Autodesk Inventor part; units mm, degrees
ref_plane "YZ Plane" through (0, 0, 0) normal (1, 0, 0) x (0, 1, 0)
ref_plane "XZ Plane" through (0, 0, 0) normal (0, 1, 0) x (-1, 0, 0)
ref_plane "XY Plane" through (0, 0, 0) normal (0, 0, 1) x (1, 0, 0)
sketch "스케치1" plane through (0, 0, 0) normal (1, 0, 0) x (0, 1, 0)
  line L0 (0, 0) -> (50, 0)
  line L1 (50, 0) -> (50, -14)
  line L2 (50, -14) -> (0, -14)
  line L3 (0, -14) -> (0, 0)
  circle A0 centre (32, -7) radius 1.5
  circle A1 centre (3, -7) radius 1.5
  line L4 (60, 16.5) -> (50, 16.5)
  line L5 (50, 16.5) -> (50, -30.5)
  line L6 (50, -30.5) -> (60, -30.5)
  line L7 (60, -30.5) -> (60, 16.5)
  circle A2 centre (55, 11.5) radius 1.5
  circle A3 centre (55, -25.5) radius 1.5
  point P0 (50, -7)
  dimension "d0" = 50
  dimension "d1" = 14
  dimension "d2" = 3
  dimension "d3" = 3
  dimension "d4" = 29
  dimension "d5" = 7
  dimension "d6" = 7
  dimension "d10" = 3
  dimension "d11" = 10
  dimension "d12" = 47
  dimension "d13" = 3
  dimension "d14" = 3
  dimension "d15" = 37
  dimension "d16" = 5
  dimension "d17" = 5
  dimension "d18" = 5
extrude "돌출2" add sketch "스케치1" along normal blind 4
sketch "스케치2" plane through (4, 0, 0) normal (1, 0, 0) x (0, 0, -1)
  circle A0 centre (7, 3) radius 1.5
  circle A1 centre (7, 32) radius 1.5
  circle A2 centre (25.5, 55) radius 1.5
  circle A3 centre (-11.5, 55) radius 1.5
  line L0 (-16.5, 50) -> (0, 50)
  line L1 (0, 50) -> (0, 0)
  line L2 (0, 0) -> (14, 0)
  line L3 (14, 0) -> (14, 50)
  line L4 (14, 50) -> (30.5, 50)
  line L5 (30.5, 50) -> (30.5, 60)
  line L6 (30.5, 60) -> (-16.5, 60)
  line L7 (-16.5, 60) -> (-16.5, 50)
  line L8 (0, 50) -> (0, 0)
  line L9 (0, 42) -> (14, 42)
  line L10 (14, 0) -> (14, 50)
  dimension "d21" = 10
bend part "굽힘1" radius 10 angle 10 line through (4, 42, 0) along (0, 0, -1) centre toward (1, 0, 0) moving side (0, 1, 0) both sides no
properties part number "옆면PSD받침대" material "ABS 플라스틱"
Geometry: final body of the model. Coordinates: model frame, mm. A direction names the side the tool comes from. Give positions to 0.01 mm unless a question says otherwise; leave off trailing zeros. Loops run counter-clockwise (first coordinate to the right, second up) from the corner with the lowest first, then second, coordinate; pieces in that order, holes last. Notation, with made-up numbers: (-10, 48) -> (39, 48) arc R29 cw to (39, 86) -> close; hole circle Ø9 at (30.25, 68.5). An arc over 180 degrees is marked (long way). Put each result on its own line as item: value.
1. Cut plane C-C (z = -1.5). Return the cut outline in (x, y), plus the area to 3 significant figures.
Taken from the geometry:
outline: (0, 0) -> (4, 0) -> (4, 42) arc R10 cw to (4.15, 43.74) -> (6.97, 59.74) -> (3.04, 60.44) -> (0.21, 44.43) arc R14 ccw to (0, 42) -> close
area: 241 mm2
2. Cut plane B-B (z = -7). Return the cut outline in (x, y), plus the area to 3 significant figures.
Taken from the geometry:
outline: (0, 0) -> (4, 0) -> (4, 1.5) -> (0, 1.5) -> close; (0, 4.5) -> (4, 4.5) -> (4, 30.5) -> (0, 30.5) -> close; (0, 33.5) -> (4, 33.5) -> (4, 42) arc R10 cw to (4.15, 43.74) -> (6.97, 59.74) -> (3.04, 60.44) -> (0.21, 44.43) arc R14 ccw to (0, 42) -> close
area: 217 mm2
3. Pull-direction query (Y, two-part tool) for faces 1 (the cylindrical face through (4.04, 42.88, -6.9)), 2 (the flat face through (4, 55, 16.5)), 3 (the cylindrical face through (4.075, 54.98, -26.987)); classes: released by +Y, released by -Y, zero draft, split by the parting line, or undercut.
Taken from the geometry:
face 1: released by -Y
face 2: zero draft
face 3: undercut
4. Set-up query: faces 4 (the flat face through (3.24, 50.25, 8.37)), 5 (the flat face through (4, 21, -7)), 6 (the flat face through (3.24, 50.25, -22.13)), 7 (the flat face through (0, 21, -7)). Return all of +Z, -Z, +X, -X, +Y, -Y with unobstructed straight access to the full face (end or side cutting, diameter ignored); none if empty.
Taken from the geometry:
face 4: +Z, -X, -Y
face 5: +Z, -Z, +X, -Y
face 6: -Z, -X, -Y
face 7: +Z, -Z, -X, +Y, -Y
5. Pin query (flat end, axial travel): P1, Ø2, axis at x = 4.5, z = 11.5, coming from the -Y side; P2, Ø5, axis at y = 3, z = -7, coming from the +X side; P3, Ø2, axis at x = 2, z = 4.5, coming from the -Y side. Return the tip coordinate at first contact, or that it passes through.
Taken from the geometry:
P1: stops at y = 49.9
P2: stops at x = 4
P3: stops at y = 50.29
6. Cut plane D-D (y = 37). Return the cut outline in (x, z), plus the area to 3 significant figures.
Taken from the geometry:
outline: (0, -14) -> (4, -14) -> (4, 0) -> (0, 0) -> close
area: 56.0 mm2
7. Cut plane A-A (y = 3). Return the cut outline in (x, z).
Taken from the geometry:
outline: (0, -14) -> (4, -14) -> (4, -8.5) -> (0, -8.5) -> close; (0, -5.5) -> (4, -5.5) -> (4, 0) -> (0, 0) -> close
8. Ray query, line 1 along Z through (x, y) = (3.15, 32); line 2 along Z through (x, y) = (3.75, 55); line 3 along X through (y, z) = (15, -4.5). Return the intervals inside material, ascending. Write a range as [from, to].
Taken from the geometry:
line 1: z = [-14, -8.5], [-5.5, 0]
line 2: z = [-30.5, -26.98], [-24.02, 10.02], [12.98, 16.5]
line 3: x = [0, 4]
